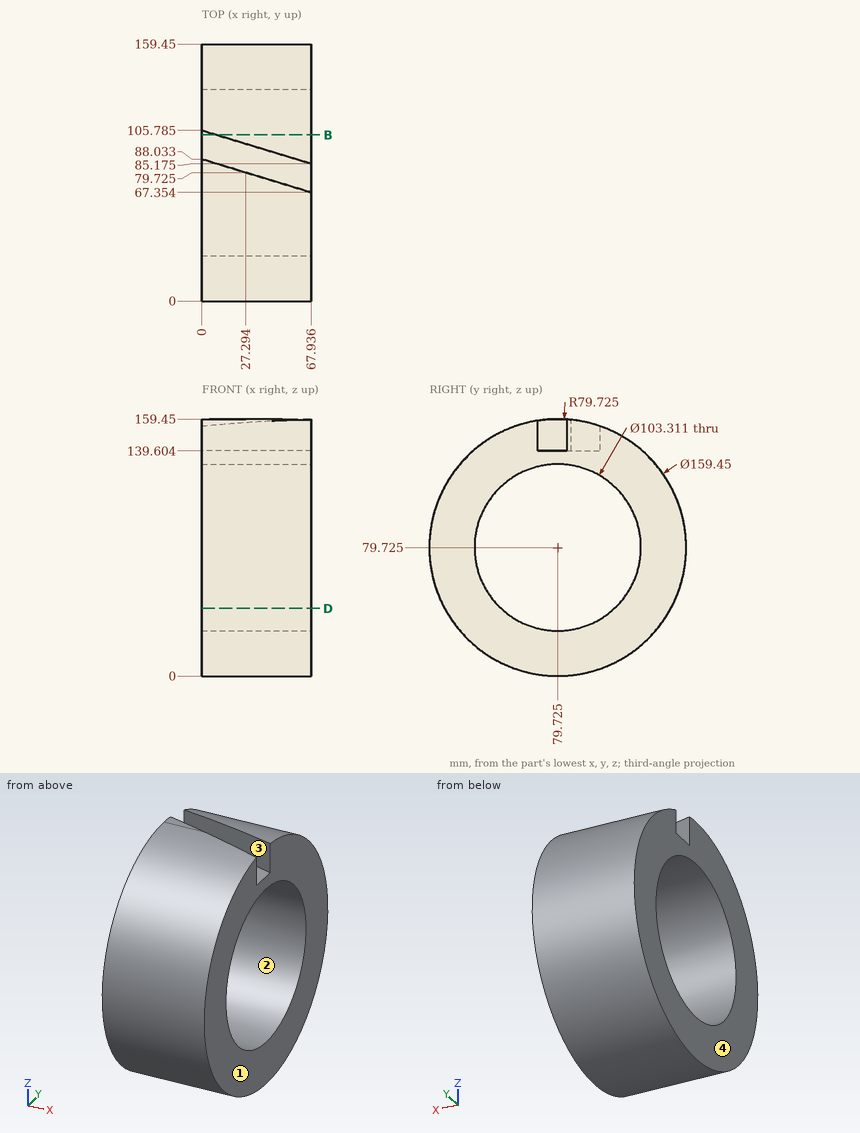
Answer from the drawing. Dimensions are ordinates in mm from the lowest x, y and z of the part. A direction names the side the tool comes from. Round coordinates to 2 decimals unless told otherwise and drop trailing zeros. Loops run counter-clockwise (first coordinate to the right, second up) from the corner with the lowest first, then second, coordinate; pieces in that order, holes last. Notation, with made-up numbers: (-22, -2.75) - (11, -2.75) arc R15 ccw to (11, 22.25) - close; hole circle Ø3 at (37, 68). An arc over 180 degrees is marked (long way). Return JSON: item names as keys, results as strings. Group by question number.
1. Each of these flat-tipped pins is pushed along its axis until it touches: P1, Ø3, axis at x = 22.5, y = 96.5, coming from the -Z side; P2, Ø1.5, axis at x = 16.5, y = 90, coming from the +Z side; P3, Ø5, axis at x = 31, y = 35.5, coming from the -Z side. Where does it stop, or does it pass through?
2. Which of the six approach directions +Z, -Z, +X, -X, +Y, -Y give full straight-line access (tool end or side, diameter ignored) to the marked faces 3 and 4?
3. The mould has two halves that part along Z. Classify the marked faces 1 and 2: pulls with the +Z half, pulls with the -Z half, needs draft (parallel to the pull), parting line crosses it, or undercut.
4. The part is cut by section B-B on y = 103. Determine the outline of the cut face in (x, z) (1 decimal).
5. Consider probe 1 along Z at (x, y) = (29.5, 50.5); probe 2 along Y at (x, z) = (43.5, 38) (1 decimal); probe 3 along Y at (x, z) = (47, 127) (1 decimal). Determine where each line is inside the solid, lowest interval first.
6. The part is cut by section D-D on z = 42. Determine the outline of the cut face in (x, y) (1 decimal).
Resolved:
{
 "1": {"P1": "stops at z = 1.48", "P2": "stops at z = 139.6", "P3": "stops at z = 11.79"},
 "2": {"face 3": "+Z", "face 4": "+Z, -Z, -X, +Y, -Y"},
 "3": {"face 1": "needs draft", "face 2": "undercut"},
 "4": {"outline": "(0, 3.5) - (67.9, 3.5) - (67.9, 33.6) - (0, 33.6) - close; (0, 125.8) - (67.9, 125.8) - (67.9, 156) - (9.2, 156) - (9.2, 139.6) - (0, 139.6) - close"},
 "5": {"probe 1": "z = 5.55 to 37.13, 122.32 to 153.9", "probe 2": "y = 11.8 to 49.3, 110.2 to 147.7", "probe 3": "y = 15.5 to 58.9, 100.5 to 143.9"},
 "6": {"outline": "(0, 9.5) - (67.9, 9.5) - (67.9, 44.4) - (0, 44.4) - close; (0, 115) - (67.9, 115) - (67.9, 150) - (0, 150) - close"}
}
